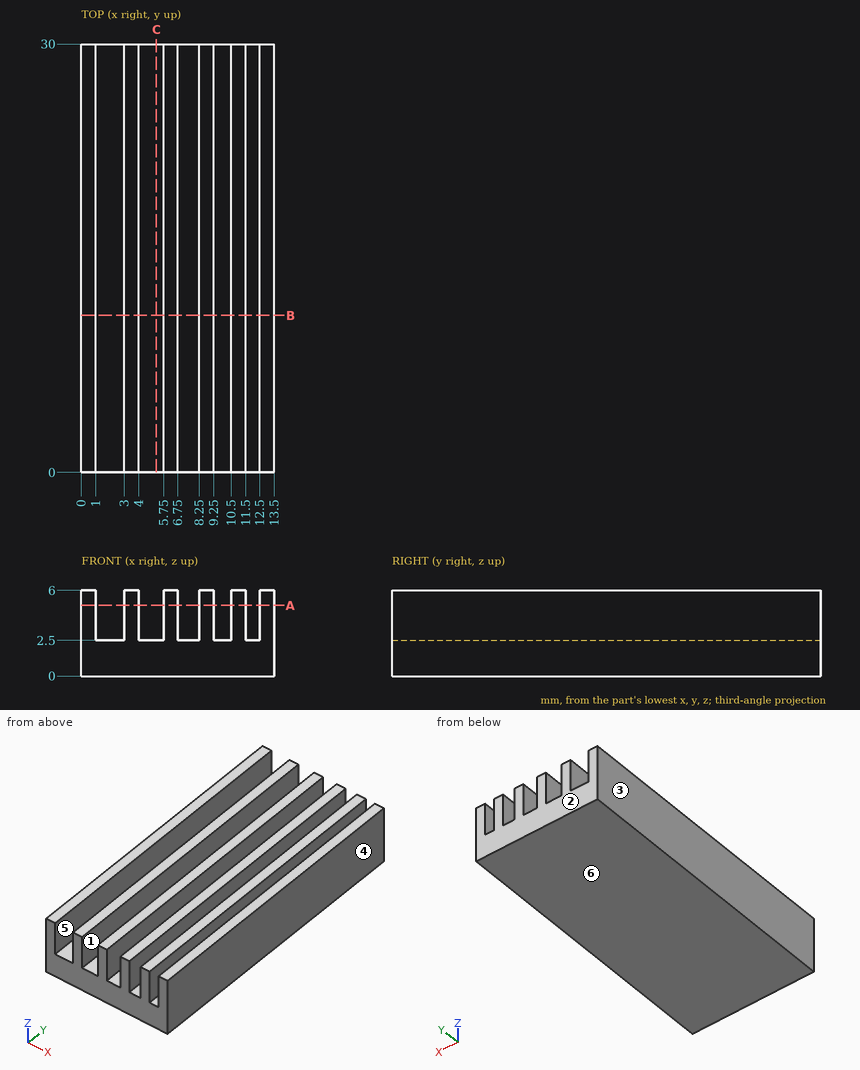
Verification items for this drawing (mm, ordinates from the low corner). A direction names the side the tool comes from. Give positions to 0.01 mm unless a question says otherwise; leave off trailing zeros. Write each loop counter-clockwise with the first axis right and the second up, starting at its lowest first coordinate (ties: lowest second). Pieces come first, ordered by that corner, then holes. Notation, with made-up numbers: (-10.75, -33.5) - (38.25, -33.5) arc R16 ccw to (38.25, -6.5) - close; hole circle Ø1 at (63, 21). An arc over 180 degrees is marked (long way). Answer as a JSON object with one key per item and string values. Group by question number.
1) Sectioned sample at B-B (y = 11). Record the cut outline in (x, z), then the cut area to 4 significant figures.
2) Sectioned sample at A-A (z = 4.95). Record the cut outline in (x, y), then the cut area to 3 significant figures.
3) Thickness scan on probe 1 along X at (y, z) = (18, 4.3); probe 2 along Z at (x, y) = (10.25, 9.5). Record the ranges inside material, lowest first. Write a range as from..to.
4) Release check for a two-part mould opening along X. For the marked faces 1, 2, 3 and 4 record: pulls with the +X half, pulls with the -X half, needs draft (parallel to the pull), parting line crosses it, or undercut.
5) Depth check by flat-ended pin: P1, Ø0.5, axis at x = 12, y = 11.5, coming from the +Z side. Enter the tip coordinate at first touch or a pass-through.
6) Access from +Z, -Z, +X, -X, +Y, -Y to the whole of each face (thin tool, end or side, straight path). Record for the marked faces 5 and 6.
7) Sectioned sample at C-C (x = 5.25). Record the cut outline in (y, z).
Geometry results:
{
 "1": {"outline": "(0, 0) - (13.5, 0) - (13.5, 6) - (12.5, 6) - (12.5, 2.5) - (11.5, 2.5) - (11.5, 6) - (10.5, 6) - (10.5, 2.5) - (9.25, 2.5) - (9.25, 6) - (8.25, 6) - (8.25, 2.5) - (6.75, 2.5) - (6.75, 6) - (5.75, 6) - (5.75, 2.5) - (4, 2.5) - (4, 6) - (3, 6) - (3, 2.5) - (1, 2.5) - (1, 6) - (0, 6) - close", "area": "54.75 mm^2"},
 "2": {"outline": "(0, 0) - (1, 0) - (1, 30) - (0, 30) - close; (3, 0) - (4, 0) - (4, 30) - (3, 30) - close; (5.75, 0) - (6.75, 0) - (6.75, 30) - (5.75, 30) - close; (8.25, 0) - (9.25, 0) - (9.25, 30) - (8.25, 30) - close; (10.5, 0) - (11.5, 0) - (11.5, 30) - (10.5, 30) - close; (12.5, 0) - (13.5, 0) - (13.5, 30) - (12.5, 30) - close", "area": "180 mm^2"},
 "3": {"probe 1": "x = 0..1, 3..4, 5.75..6.75, 8.25..9.25, 10.5..11.5, 12.5..13.5", "probe 2": "z = 0..2.5"},
 "4": {"face 1": "undercut", "face 2": "needs draft", "face 3": "pulls with the -X half", "face 4": "pulls with the +X half"},
 "5": {"P1": "stops at z = 2.5"},
 "6": {"face 5": "+Z, +Y, -Y", "face 6": "-Z, +X, -X, +Y, -Y"},
 "7": {"outline": "(0, 0) - (30, 0) - (30, 2.5) - (0, 2.5) - close"}
}
